Design review of the part shown in the three views and the two pictorial views. Dimensions are in mm from the part's minimum x, y and z. A direction names the side the tool comes from. Give positions to 0.01 mm unless a question says otherwise; leave off trailing zeros. Order: outer loops, then holes, each group sorted by start corner. A loop starts at its lowest first (then second) coordinate and runs counter-clockwise, first axis right, second up.
Item 1: Consider section A-A (y = 13.5). Give the boundary of the cut face in (x, z).
Item 2: Consider section B-B (x = 20). Give the boundary of the cut face in (y, z).
Item 3: For P1, Ø1, axis at x = 16.5, z = 3.5, coming from the +Y side; P2, Ø1, axis at x = 4.5, y = 12, coming from the +Z side; P3, Ø3, axis at x = 14, z = 2, coming from the +Y side (3 decimals), all flat-tipped, find the tip position at first contact; note any pin that passes through.
Item 4: Machinability: for the marked faces 1, 2, 3 and 4, which of the approach directions +Z, -Z, +X, -X, +Y, -Y give a long, thin tool a straight path to every point of the face, cutting with its end or side? Answer none if there is none.
Item 5: Consider section D-D (x = 4). Give the boundary of the cut face in (y, z).
Item 6: For probe 1 along X at (y, z) = (20, 3); probe 2 along Z at (x, y) = (21, 43); probe 3 along Y at (x, z) = (26.5, 6), list the stretches that pass through material, from the lowest coordinate up.
Item 7: Consider section C-C (z = 8.5). Give the boundary of the cut face in (x, y).
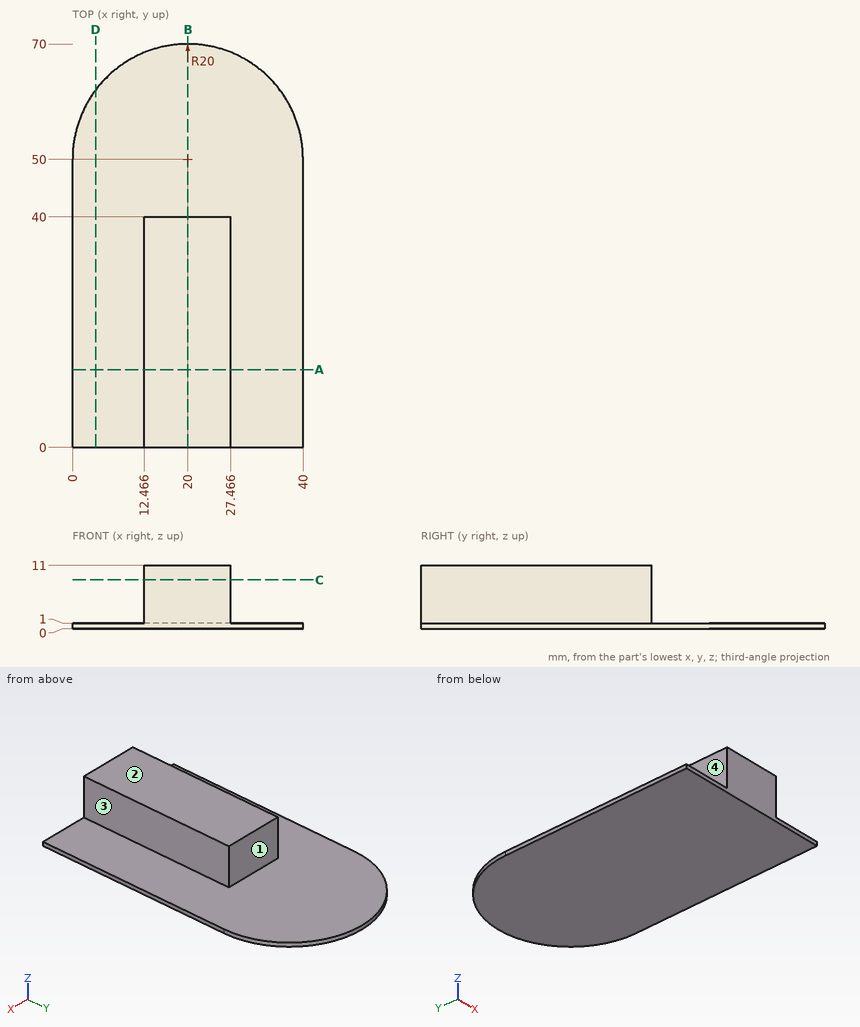
Resolved:
1. outline: (0, 0) - (40, 0) - (40, 1) - (27.47, 1) - (27.47, 11) - (12.47, 11) - (12.47, 1) - (0, 1) - close
2. outline: (0, 0) - (70, 0) - (70, 1) - (40, 1) - (40, 11) - (0, 11) - close
3. P1: stops at y = 40
3. P2: stops at z = 1
3. P3: stops at y = 69.395
4. face 1: +Z, +X, -X, +Y
4. face 2: +Z, +X, -X, +Y, -Y
4. face 3: +Z, +X, +Y, -Y
4. face 4: +Z, -X, +Y, -Y
5. outline: (0, 0) - (62, 0) - (62, 1) - (0, 1) - close
6. probe 1: x = 12.47 to 27.47
6. probe 2: z = 0 to 1
6. probe 3: y = 0 to 40
7. outline: (12.47, 0) - (27.47, 0) - (27.47, 40) - (12.47, 40) - close
